Job drawing, mm, ordinate dimensions from the low corner. One solid piece. A direction names the side the tool comes from. Coordinates: 2 decimals unless noted, no trailing zeros. Loops run counter-clockwise (first coordinate to the right, second up) from the corner with the lowest first, then second, coordinate; pieces in that order, holes last. Notation, with made-up numbers: (80, 48.5) -> (106, 48.5) arc R24 cw to (106, 72.5) -> close; hole circle Ø4 at (47, 44.5). An arc over 180 degrees is marked (long way). Answer as CSV lines item,"result". Start each with the question number.
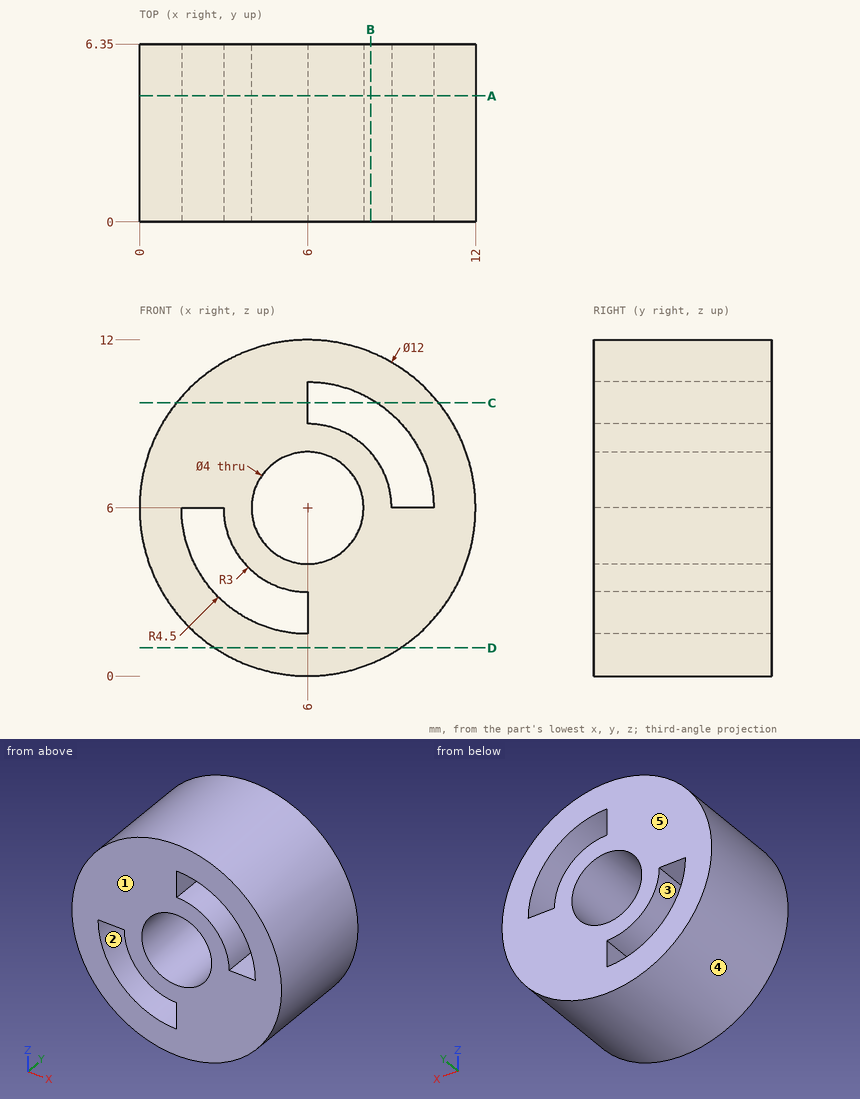
Q1. Probe probe 1 along Z at (x, y) = (7.75, 5); probe 2 along X at (y, z) = (4.75, 4.5); probe 3 along Z at (x, y) = (5.5, 3.5). List the from-to ranges inside material, lowest first. Write a range as from..to.
Q2. Saw through at A-A (y = 4.5). List the corners of the cut face in (x, z), and give its area (3 significant figures).
Q3. Two-plate mould, pull along Z, no slides. Class the marked faces 3, 4 and 5: pulls with the +Z half, pulls with the -Z half, needs draft (parallel to the pull), parting line crosses it, or undercut.
Q4. Which spindle directions (+Z, -Z, +X, -X, +Y, -Y) get a long thin tool onto all of the face, cutting with end or side? Do the marked faces 1 and 2. Say none if no direction does.
Q5. Pin check, flat tips, straight feed: pin 1 Ø2 at (x, y) = (2.5, 1) entering from -Z; pin 2 Ø3 at (x, z) = (6, 6) entering from -Y; pin 3 Ø0.8 at (y, z) = (3.5, 9.5) entering from +X; pin 4 Ø3 at (x, y) = (10, 2.5) entering from +Z. Stop position of each tip, or through.
Q6. Saw through at D-D (z = 1). List the corners of the cut face in (x, y), and give its area (3 significant figures).
Q7. Saw through at C-C (z = 9.75). List the corners of the cut face in (x, y).
Q8. Saw through at B-B (x = 8.25). List the corners of the cut face in (y, z).
Ans:
1,probe 1,"z = 0.26..5.03, 6.97..8.44, 10.15..11.74"
1,probe 2,"x = 0.19..1.76, 3.4..4.68, 7.32..11.81"
1,probe 3,"z = 0.02..1.53, 3.04..4.06, 7.94..11.98"
2,outline,"circle Ø12 at (6, 6); hole (1.5, 6) arc R4.5 ccw to (6, 1.5) -> (6, 3) arc R3 cw to (3, 6) -> close; hole circle Ø4 at (6, 6); hole (6, 9) arc R3 cw to (9, 6) -> (10.5, 6) arc R4.5 ccw to (6, 10.5) -> close"
2,area,"82.9 mm²"
3,face 3,"undercut"
3,face 4,"parting line crosses it"
3,face 5,"needs draft"
4,face 1,"+Z, -Z, +X, -X, -Y"
4,face 2,"+Y, -Y"
5,pin 1,"stops at z = 0.55"
5,pin 2,"passes through"
5,pin 3,"stops at x = 11.14"
5,pin 4,"stops at z = 11.45"
6,outline,"(2.68, 0) -> (9.32, 0) -> (9.32, 6.35) -> (2.68, 6.35) -> close"
6,area,"42.1 mm²"
7,outline,"(1.32, 0) -> (6, 0) -> (6, 6.35) -> (1.32, 6.35) -> close; (8.49, 0) -> (10.68, 0) -> (10.68, 6.35) -> (8.49, 6.35) -> close"
8,outline,"(0, 0.44) -> (6.35, 0.44) -> (6.35, 7.98) -> (0, 7.98) -> close; (0, 9.9) -> (6.35, 9.9) -> (6.35, 11.56) -> (0, 11.56) -> close"
